```python
from build123d import *

# Parameters (mm, degrees)
SKETCH1_W           = 39
SKETCH1_H           = 39
BOSS_EXTRUDE1_DEPTH = 14
FILLET1_R           = 2
FILLET2_R           = 2
SKETCH2_W           = 8
SKETCH2_H           = 18
SKETCH2_W_2         = 1.12294134
SKETCH2_H_2         = 1.122941341
CUT_EXTRUDE1_DEPTH  = 4
SKETCH2_2_W         = 1.12294134
SKETCH2_2_H         = 1.122941341
BOSS_EXTRUDE3_DEPTH = 4
SKETCH3_W           = 7
SKETCH3_H           = 3
CUT_EXTRUDE2_DEPTH  = 2


with BuildPart() as part:
    # Sketch1 → Boss-Extrude1 (new body)
    with BuildSketch(Plane(origin=(0, 0, 0), x_dir=(1, 0, 0), z_dir=(0, 1, 0))):
        Rectangle(SKETCH1_W, SKETCH1_H)
    extrude(amount=BOSS_EXTRUDE1_DEPTH)

    # Fillet1
    fillet1_edges = [part.edges().sort_by_distance(p)[0] for p in [
        (19.5, 7, 19.5),
        (-19.5, 7, 19.5),
        (-19.5, 7, -19.5),
        (19.5, 7, -19.5),
    ]]
    fillet(fillet1_edges, radius=FILLET1_R)

    # Fillet2
    fillet2_edges = [part.edges().sort_by_distance(p)[0] for p in [
        (0, 14, 19.5),
        (-19.5, 14, 0),
        (19.5, 14, 0),
        (0, 14, -19.5),
        (18.914213562, 14, 18.914213562),
        (18.914213562, 14, -18.914213562),
        (-18.914213562, 14, -18.914213562),
        (-18.914213562, 14, 18.914213562),
    ]]
    fillet(fillet2_edges, radius=FILLET2_R)

    # Sketch2 → Cut-Extrude1 (cut)
    with BuildSketch(Plane(origin=(0, 14, 0), x_dir=(1, 0, 0), z_dir=(0, 1, 0))):
        with Locations((13.5, 4.220700243)):
            Rectangle(SKETCH2_W, SKETCH2_H)
        with Locations((13.54, 11.720700244)):
            Rectangle(SKETCH2_W_2, SKETCH2_H_2, mode=Mode.SUBTRACT)
        with Locations((11, 11.720700244)):
            Rectangle(SKETCH2_W_2, SKETCH2_H_2, mode=Mode.SUBTRACT)
        with Locations((16.08, 11.720700244)):
            Rectangle(SKETCH2_W_2, SKETCH2_H_2, mode=Mode.SUBTRACT)
        with Locations((11, 8.720700244)):
            Rectangle(SKETCH2_W_2, SKETCH2_H_2, mode=Mode.SUBTRACT)
        with Locations((13.54, 8.720700244)):
            Rectangle(SKETCH2_W_2, SKETCH2_H_2, mode=Mode.SUBTRACT)
        with Locations((16.08, 8.720700244)):
            Rectangle(SKETCH2_W_2, SKETCH2_H_2, mode=Mode.SUBTRACT)
        with Locations((11, 5.720700244)):
            Rectangle(SKETCH2_W_2, SKETCH2_H_2, mode=Mode.SUBTRACT)
        with Locations((13.54, 5.720700244)):
            Rectangle(SKETCH2_W_2, SKETCH2_H_2, mode=Mode.SUBTRACT)
        with Locations((16.08, 5.720700244)):
            Rectangle(SKETCH2_W_2, SKETCH2_H_2, mode=Mode.SUBTRACT)
        with Locations((11, 2.720700244)):
            Rectangle(SKETCH2_W_2, SKETCH2_H_2, mode=Mode.SUBTRACT)
        with Locations((13.54, 2.720700244)):
            Rectangle(SKETCH2_W_2, SKETCH2_H_2, mode=Mode.SUBTRACT)
        with Locations((16.08, 2.720700244)):
            Rectangle(SKETCH2_W_2, SKETCH2_H_2, mode=Mode.SUBTRACT)
        with Locations((11, -0.279299757)):
            Rectangle(SKETCH2_W_2, SKETCH2_H_2, mode=Mode.SUBTRACT)
        with Locations((13.54, -0.279299757)):
            Rectangle(SKETCH2_W_2, SKETCH2_H_2, mode=Mode.SUBTRACT)
        with Locations((16.08, -0.279299757)):
            Rectangle(SKETCH2_W_2, SKETCH2_H_2, mode=Mode.SUBTRACT)
        with Locations((11, -3.279299757)):
            Rectangle(SKETCH2_W_2, SKETCH2_H_2, mode=Mode.SUBTRACT)
        with Locations((13.54, -3.279299757)):
            Rectangle(SKETCH2_W_2, SKETCH2_H_2, mode=Mode.SUBTRACT)
        with Locations((16.08, -3.279299757)):
            Rectangle(SKETCH2_W_2, SKETCH2_H_2, mode=Mode.SUBTRACT)
    extrude(amount=-CUT_EXTRUDE1_DEPTH, mode=Mode.SUBTRACT)

    # Sketch2<2> → Boss-Extrude3 (add)
    with BuildSketch(Plane(origin=(0, 14, 0), x_dir=(1, 0, 0), z_dir=(0, 1, 0))):
        with Locations((13.54, 11.720700244)):
            Rectangle(SKETCH2_2_W, SKETCH2_2_H)
        with Locations((11, 11.720700244)):
            Rectangle(SKETCH2_2_W, SKETCH2_2_H)
        with Locations((16.08, 11.720700244)):
            Rectangle(SKETCH2_2_W, SKETCH2_2_H)
        with Locations((11, 8.720700244)):
            Rectangle(SKETCH2_2_W, SKETCH2_2_H)
        with Locations((13.54, 8.720700244)):
            Rectangle(SKETCH2_2_W, SKETCH2_2_H)
        with Locations((16.08, 8.720700244)):
            Rectangle(SKETCH2_2_W, SKETCH2_2_H)
        with Locations((11, 5.720700244)):
            Rectangle(SKETCH2_2_W, SKETCH2_2_H)
        with Locations((13.54, 5.720700244)):
            Rectangle(SKETCH2_2_W, SKETCH2_2_H)
        with Locations((16.08, 5.720700244)):
            Rectangle(SKETCH2_2_W, SKETCH2_2_H)
        with Locations((11, 2.720700244)):
            Rectangle(SKETCH2_2_W, SKETCH2_2_H)
        with Locations((13.54, 2.720700244)):
            Rectangle(SKETCH2_2_W, SKETCH2_2_H)
        with Locations((16.08, 2.720700244)):
            Rectangle(SKETCH2_2_W, SKETCH2_2_H)
        with Locations((11, -0.279299757)):
            Rectangle(SKETCH2_2_W, SKETCH2_2_H)
        with Locations((13.54, -0.279299757)):
            Rectangle(SKETCH2_2_W, SKETCH2_2_H)
        with Locations((16.08, -0.279299757)):
            Rectangle(SKETCH2_2_W, SKETCH2_2_H)
        with Locations((11, -3.279299757)):
            Rectangle(SKETCH2_2_W, SKETCH2_2_H)
        with Locations((13.54, -3.279299757)):
            Rectangle(SKETCH2_2_W, SKETCH2_2_H)
        with Locations((16.08, -3.279299757)):
            Rectangle(SKETCH2_2_W, SKETCH2_2_H)
    extrude(amount=BOSS_EXTRUDE3_DEPTH)

    # Sketch3 → Cut-Extrude2 (cut)
    with BuildSketch(Plane.ZY.offset(19.5)):
        with Locations((-0.380147746, 10.5)):
            Rectangle(SKETCH3_W, SKETCH3_H)
    extrude(amount=-CUT_EXTRUDE2_DEPTH, mode=Mode.SUBTRACT)


solid = part.part
```
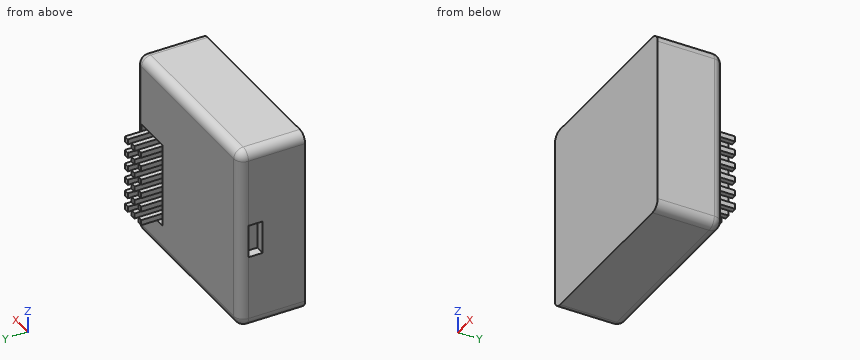
The model under review builds one solid part; all positions refer to its coordinate system, in mm. Give positions to 0.01 mm unless a question says otherwise; leave off trailing zeros. Write each loop counter-clockwise with the first axis right and the second up, starting at its lowest first coordinate (ties: lowest second). Pieces come first, ordered by that corner, then holes. Notation, with made-up numbers: (75.25, 23.5) - (81.25, 23.5) arc R22 ccw to (81.25, 40.5) - close; hole circle Ø7 at (2, 23). An arc over 180 degrees is marked (long way). Answer in a Markdown table with one row per item. Add a question column.
1. We need section A-A on y = 11.25. State how many separate pieces and enclosed holes the cut face has, then the cut area to 3 significant figures.
2. Insertion check: P1, Ø5, axis at x = 10.5, z = 8, coming from the +Y side; P2, Ø1.2, axis at x = 11, y = 14, coming from the -Z side; P3, Ø3, axis at y = 16, z = -13.5, coming from the -X side. Each pin has a flat end and moves straight along its axis. Give the tip position at first contact, or say it passes through.
3. Wall thickness on line 1 along Y through (x, z) = (3, 17); line 2 along X through (y, z) = (13, -1.5); line 3 along Z through (x, y) = (-4, 12.5): over which ranges is each line inside the solid? List them lowest first. Write a range as [from, to].
4. We need section D-D on z = 10. Write out the cut boundary in (x, y), then the cut area to 3 significant figures.
Ans:
| question | item | result |
|---|---|---|
| 1 | separate pieces | 19 |
| 1 | enclosed holes | 1 |
| 1 | area | 1,380 mm^2 |
| 2 | P1 | stops at y = 14 |
| 2 | P2 | stops at z = -18.93 |
| 2 | P3 | stops at x = 10.44 |
| 3 | line 1 | y = [0, 14] |
| 3 | line 2 | x = [-19.23, 9.5], [17.5, 19.23] |
| 3 | line 3 | z = [-19.44, 19.44] |
| 4 | outline | (-19.5, 0) - (19.5, 0) - (19.5, 12) arc R2 ccw to (17.5, 14) - (-17.5, 14) arc R2 ccw to (-19.5, 12) - close |
| 4 | area | 544 mm^2 |
